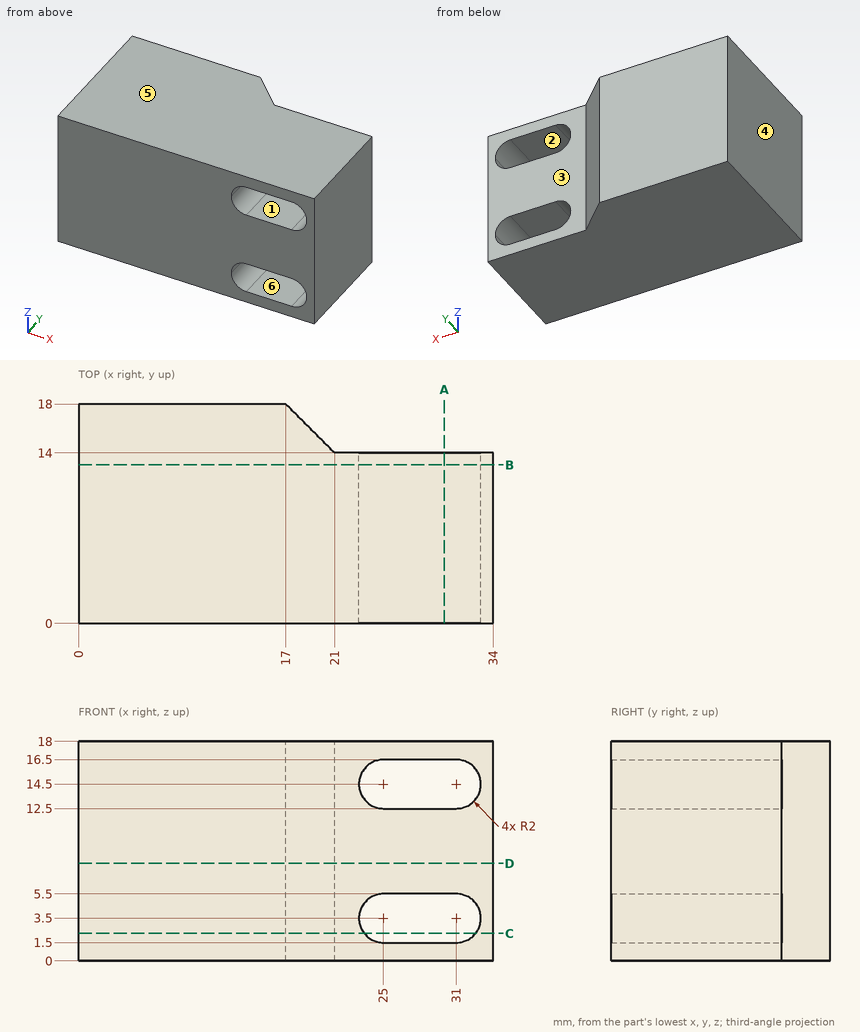
The figure shows three views and two pictorial views of one solid part (mm, origin at its lowest corner). Answer the questions. A direction names the side the tool comes from. Coordinates: 2 decimals unless noted, no trailing zeros. Write each loop counter-clockwise with the first axis right and the second up, starting at its lowest first coordinate (ties: lowest second). Pieces come first, ordered by that corner, then holes. Notation, with made-up numbers: M 0.5,-5.75 L 52.5,-5.75 A16 cw 52.5,5.25 Z; hole C 37,80.5 d1. An arc over 180 degrees is marked long. Answer as CSV lines item,"result". Start each with the question number.
Item 1: Consider L1, parallel to Z at x = 25.5, y = 3; L2, parallel to Y at x = 22, z = 15.75; L3, parallel to X at y = 6.5, z = 13.5. Determine where each line is inside the solid, lowest interval first.
Item 2: Section C-C on z = 2.25 is taken. Write down the section's boundary in (x, y), and give its area (3 significant figures).
Item 3: Section A-A on x = 30 is taken. Write down the section's boundary in (y, z).
Item 4: A tool of negligible diameter and unlimited length cuts with its end or side. For the marked faces 5 and 6, from which of +Z, -Z, +X, -X, +Y, -Y can it reach the whole face along a straight path? Write none if from no direction.
Item 5: Determine the mould class of the marked faces 1, 2, 3 and 4 for opening direction X: released by +X, released by -X, zero draft, split by the parting line, or undercut.
Item 6: Flat-ended cylindrical pins translate along their axes: P1, Ø5, axis at x = 26.5, z = 4.5, coming from the +Y side; P2, Ø1.8, axis at x = 27, y = 8, coming from the -Z side. Find the tip coordinate at first contact, or state that the pin passes through.
Item 7: Section D-D on z = 8 is taken. Write down the section's boundary in (x, y).
Item 8: Section B-B on y = 13 is taken. Write down the section's boundary in (x, z), and give its area (3 significant figures).
Checks:
1,L1,"z = 0 to 1.5, 5.5 to 12.5, 16.5 to 18"
1,L2,"y = 0 to 14"
1,L3,"x = 0 to 23.27, 32.73 to 34"
2,outline,"M 0,0 L 23.44,0 L 23.44,14 L 21,14 L 17,18 L 0,18 Z; M 32.56,0 L 34,0 L 34,14 L 32.56,14 Z"
2,area,"424 mm²"
3,outline,"M 0,0 L 14,0 L 14,1.5 L 0,1.5 Z; M 0,5.5 L 14,5.5 L 14,12.5 L 0,12.5 Z; M 0,16.5 L 14,16.5 L 14,18 L 0,18 Z"
4,face 5,"+Z, +X, -X, +Y, -Y"
4,face 6,"+Y, -Y"
5,face 1,"undercut"
5,face 2,"undercut"
5,face 3,"zero draft"
5,face 4,"released by -X"
6,P1,"stops at y = 14"
6,P2,"stops at z = 0"
7,outline,"M 0,0 L 34,0 L 34,14 L 21,14 L 17,18 L 0,18 Z"
8,outline,"M 0,0 L 34,0 L 34,18 L 0,18 Z; hole M 23,3.5 A2 ccw 25,1.5 L 31,1.5 A2 ccw 33,3.5 A2 ccw 31,5.5 L 25,5.5 A2 ccw Z; hole M 23,14.5 A2 ccw 25,12.5 L 31,12.5 A2 ccw 33,14.5 A2 ccw 31,16.5 L 25,16.5 A2 ccw Z"
8,area,"539 mm²"
